For this review, take the finished solid that the model builds, in its own axes (mm). A direction names the side the tool comes from. Round coordinates to 2 decimals unless told otherwise and drop trailing zeros. Order: outer loops, then holes, each group sorted by start corner. A loop starts at its lowest first (then second) coordinate and runs counter-clockwise, first axis right, second up. Notation, with made-up numbers: (44, -23) -> (68, -23) arc R15 cw to (68, -15) -> close; hole circle Ø6 at (-25, 10.25). An arc over 180 degrees is marked (long way). Put each result on its own line as item: value. Start each with the question number.
```python
from build123d import *

# Parameters (mm, degrees)
F0_W     = 40
F0_H     = 12
F0_R     = 2.75
F1_DEPTH = 5
F2_W     = 40
F2_H     = 10
F2_H_2   = 5
F3_DEPTH = 5
F4_W     = 40
F4_H     = 5
F5_DEPTH = 38
F6_W     = 20
F6_H     = 10
F7_DEPTH = 1.2
F8_R     = 1
F9_DEPTH = 25


with BuildPart() as f1:
    # F0 (on Front) → F1 (new body)
    with BuildSketch(Plane.XZ):
        with Locations((20, 6)):
            Rectangle(F0_W, F0_H)
        with Locations((10, 6)):
            Circle(F0_R, mode=Mode.SUBTRACT)
        with Locations((30, 6)):
            Circle(F0_R, mode=Mode.SUBTRACT)
    extrude(amount=F1_DEPTH)

    # F2 (on face) → F3 (join)
    with BuildSketch(Plane(origin=(0, 0, 0), x_dir=(1, 0, 0), z_dir=(0, 0, -1))):
        with Locations((20, -5)):
            Rectangle(F2_W, F2_H)
        with Locations((20, 2.5)):
            Rectangle(F2_W, F2_H_2)
    extrude(amount=F3_DEPTH)

    # F4 (on face) → F5 (join)
    with BuildSketch(Plane(origin=(0, 0, -5), x_dir=(1, 0, 0), z_dir=(0, 0, -1))):
        with Locations((20, -7.5)):
            Rectangle(F4_W, F4_H)
    extrude(amount=F5_DEPTH)

    # F6 (on face) → F7 (cut)
    with BuildSketch(Plane.XZ.offset(-5)):
        with Locations((20, -38)):
            Rectangle(F6_W, F6_H)
    extrude(amount=-F7_DEPTH, mode=Mode.SUBTRACT)

    # F8 (on face) → F9 (cut)
    with BuildSketch(Plane.XZ.offset(-6.2)):
        with Locations((15, -35.5)):
            Circle(F8_R)
        with Locations((25, -35.5)):
            Circle(F8_R)
    extrude(amount=-F9_DEPTH, mode=Mode.SUBTRACT)


solid = f1.part
```
Item 1: Tool access review of faces 4 (the face through (20, 0, -5)), 5 (the face through (20, 5, 0)), 6 (the face through (20, 6, -33)): name each direction out of +Z, -Z, +X, -X, +Y, -Y from which nothing blocks a thin tool from reaching the whole face with its end or side.
Item 2: Consider section B-B, the plane x = 15. Write out the cut boundary in (y, z), plus the area to 3 significant figures.
Item 3: Consider section D-D, the plane y = -1.5. Write out the cut boundary in (x, z).
Item 4: Mouldability with a two-part tool opening along X and no side actions: class faces 1 (the face through (0, 6, -15)), 2 (the face through (30, 6, -38)), 3 (the face through (20, 10, -21)) as +X half, -X half, draft (parallel to the pull), parting line (faces both ways), or undercut.
Item 5: Consider section C-C, the plane x = 19.5. Write out the cut boundary in (y, z).
Item 6: For L1, parallel to Z at x = 30, y = -2.4; L2, parallel to X at y = -3.5, z = 5; L3, parallel to Y at x = 34, z = 4, list the stretches that pass through material, from the lowest coordinate up.
Item 7: Consider section A-A, the plane z = -35.5. Write out the cut boundary in (x, y).
Item 8: Insertion check: pin 1 Ø0.6 at (y, z) = (6, -40.5) entering from -X; pin 2 Ø7 at (x, z) = (10, 6) entering from +Y; pin 3 Ø3.5 at (x, z) = (30, 6) entering from -Y; pin 4 Ø8 at (x, y) = (14, 7.5) entering from +Z. Each pin has a flat end and moves straight along its axis. Give the tip position at first contact, or say it passes through.
Evaluation:
1. face 4: -Z, +X, -X, -Y
1. face 5: +Z, +X, -X, +Y
1. face 6: -Z, -Y
2. outline: (-5, -5) -> (5, -5) -> (5, -33) -> (6.2, -33) -> (6.2, -34.5) -> (10, -34.5) -> (10, 0) -> (0, 0) -> (0, 12) -> (-5, 12) -> close; (6.2, -43) -> (10, -43) -> (10, -36.5) -> (6.2, -36.5) -> close
2. area: 305 mm^2
3. outline: (0, -5) -> (40, -5) -> (40, 12) -> (0, 12) -> close; hole circle Ø5.5 at (10, 6); hole circle Ø5.5 at (30, 6)
4. face 1: -X half
4. face 2: undercut
4. face 3: draft
5. outline: (-5, -5) -> (5, -5) -> (5, -33) -> (6.2, -33) -> (6.2, -43) -> (10, -43) -> (10, 0) -> (0, 0) -> (0, 12) -> (-5, 12) -> close
6. L1: z = -5 to 3.25, 8.75 to 12
6. L2: x = 0 to 7.44, 12.56 to 27.44, 32.56 to 40
6. L3: y = -5 to 0
7. outline: (0, 5) -> (10, 5) -> (10, 6.2) -> (14, 6.2) -> (14, 10) -> (0, 10) -> close; (16, 6.2) -> (24, 6.2) -> (24, 10) -> (16, 10) -> close; (26, 6.2) -> (30, 6.2) -> (30, 5) -> (40, 5) -> (40, 10) -> (26, 10) -> close
8. pin 1: stops at x = 0
8. pin 2: stops at y = 0
8. pin 3: passes through
8. pin 4: stops at z = 0
